Check sheet for the modelled part. Datum: model origin and axes. Units: mm. A direction names the side the tool comes from. Round coordinates to 2 decimals unless told otherwise and drop trailing zeros. Order: outer loops, then holes, each group sorted by start corner. A loop starts at its lowest first (then second) coordinate and runs counter-clockwise, first axis right, second up.
```python
from build123d import *

# Parameters (mm, degrees)
SKETCH1_W           = 42.418
SKETCH1_H           = 42.418
SKETCH1_R           = 1.5494
SKETCH1_R_2         = 13.462
BOSS_EXTRUDE1_DEPTH = 3.175
SKETCH3_W           = 42.418
SKETCH3_H           = 4.191
BOSS_EXTRUDE2_DEPTH = 37.465


with BuildPart() as part:
    # Sketch1 → Boss-Extrude1 (new body)
    with BuildSketch(Plane(origin=(0, 0, 0), x_dir=(1, 0, 0), z_dir=(0, 1, 0))):
        Rectangle(SKETCH1_W, SKETCH1_H)
        with Locations((15.494, 15.494)):
            Circle(SKETCH1_R, mode=Mode.SUBTRACT)
        with Locations((-15.494, 15.494)):
            Circle(SKETCH1_R, mode=Mode.SUBTRACT)
        with Locations((15.494, -15.494)):
            Circle(SKETCH1_R, mode=Mode.SUBTRACT)
        with Locations((-15.494, -15.494)):
            Circle(SKETCH1_R, mode=Mode.SUBTRACT)
        Circle(SKETCH1_R_2, mode=Mode.SUBTRACT)
    extrude(amount=BOSS_EXTRUDE1_DEPTH)

    # Sketch3 → Boss-Extrude2 (add)
    with BuildSketch(Plane(origin=(0, 3.175, 0), x_dir=(1, 0, 0), z_dir=(0, 1, 0))):
        with Locations((0, 23.3045)):
            Rectangle(SKETCH3_W, SKETCH3_H)
    extrude(amount=-BOSS_EXTRUDE2_DEPTH)


solid = part.part
```
Item 1: Release check for a two-part mould opening along X. For faces 3 (the cylindrical face through (-10.683, 1.565, 8.191)), 4 (the flat face through (-21.209, 1, -12)), 5 (the flat face through (0, -34.29, -23)) record: released by +X, released by -X, zero draft, split by the parting line, or undercut.
Answer:
face 3: undercut
face 4: released by -X
face 5: zero draft
Item 2: Sectioned sample at D-D (x = 4.5). Record the cut outline in (y, z) (3 decimals).
Answer:
outline: (-34.29, -25.4) - (3.175, -25.4) - (3.175, -12.688) - (0, -12.688) - (0, -21.209) - (-34.29, -21.209) - close; (0, 12.688) - (3.175, 12.688) - (3.175, 21.209) - (0, 21.209) - close
Item 3: Sectioned sample at C-C (z = -10.5). Record the cut outline in (x, y) (3 decimals), and give its area (3 significant figures).
Answer:
outline: (-21.209, 0) - (-8.425, 0) - (-8.425, 3.175) - (-21.209, 3.175) - close; (8.425, 0) - (21.209, 0) - (21.209, 3.175) - (8.425, 3.175) - close
area: 81.2 mm2
Item 4: Access from +Z, -Z, +X, -X, +Y, -Y to the whole of each face (thin tool, end or side, straight path). Record for faces 1 (the flat face through (0, -17, -21.209)), 2 (the cylindrical face through (-16.64, 1.57, 14.45)).
Answer:
face 1: +Z, +X, -X, -Y
face 2: +Y, -Y
Item 5: Sectioned sample at A-A (x = 0). Record the cut outline in (y, z) (3 decimals), and give its area (3 significant figures).
Answer:
outline: (-34.29, -25.4) - (3.175, -25.4) - (3.175, -13.462) - (0, -13.462) - (0, -21.209) - (-34.29, -21.209) - close; (0, 13.462) - (3.175, 13.462) - (3.175, 21.209) - (0, 21.209) - close
area: 206 mm2
Item 6: Sectioned sample at B-B (z = 0). Record the cut outline in (x, y) (3 decimals).
Answer:
outline: (-21.209, 0) - (-13.462, 0) - (-13.462, 3.175) - (-21.209, 3.175) - close; (13.462, 0) - (21.209, 0) - (21.209, 3.175) - (13.462, 3.175) - close
Item 7: Scan lines: line 1 along X through (y, z) = (2.2, 0); line 2 along Z through (x, y) = (-13, -2); line 3 along Y through (x, z) = (-10.5, -12.5) (3 decimals). Record each from-to range of solid material in increasing order.
Answer:
line 1: x = -21.21 to -13.46, 13.46 to 21.21
line 2: z = -25.4 to -21.21
line 3: y = 0 to 3.175
Item 8: Go/stop test with flat-tipped pins: P1, Ø10.5, axis at x = -5.5, y = -11.5, coming from the +Z side; P2, Ø4, axis at x = 15.494, z = -15.494, coming from the -Y side. Record where each tip stops, or that it passes through.
Answer:
P1: stops at z = -21.21
P2: stops at y = 0
